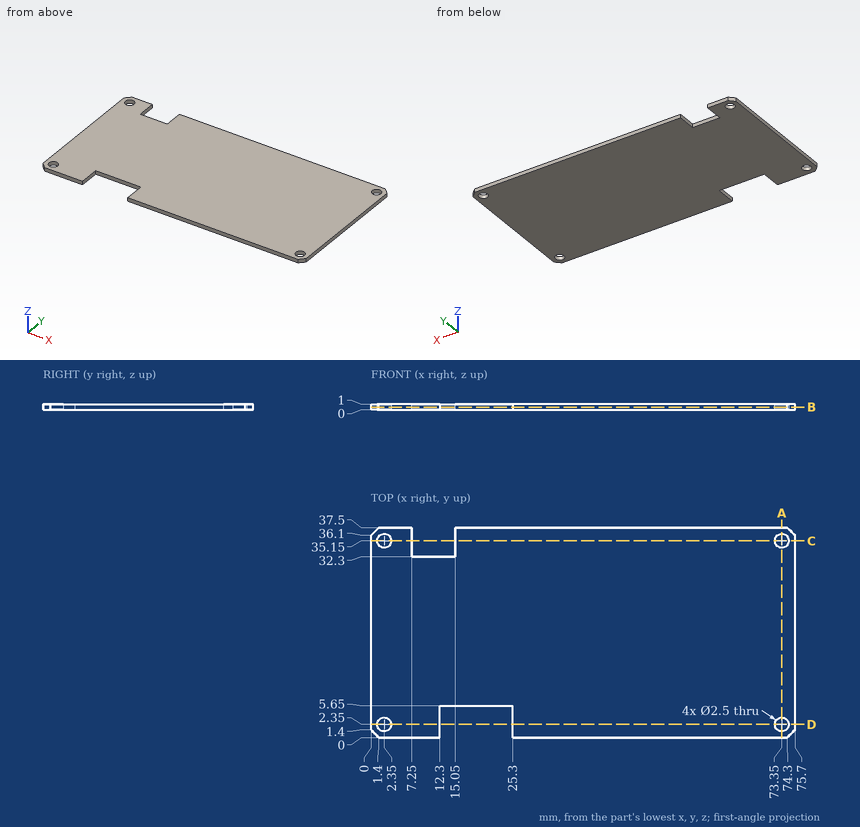
Verification items for this drawing (mm, ordinates from the low corner). Give positions to 0.01 mm unless a question says otherwise; leave off trailing zeros. Loops run counter-clockwise (first coordinate to the right, second up) from the corner with the lowest first, then second, coordinate; pieces in that order, holes last.
(1) Section check D-D on y = 2.35. Record the cut outline in (x, z).
From the geometry:
outline: (0, 0) - (1.1, 0) - (1.1, 1) - (0, 1) - close; (3.6, 0) - (12.3, 0) - (12.3, 1) - (3.6, 1) - close; (25.3, 0) - (72.1, 0) - (72.1, 1) - (25.3, 1) - close; (74.6, 0) - (75.7, 0) - (75.7, 1) - (74.6, 1) - close
(2) Depth check by flat-ended pin: pin 1 Ø10 at (x, y) = (54.5, 21.5) entering from -Z; pin 2 Ø0.5 at (x, z) = (9.5, 0.5) entering from +Y; pin 3 Ø1.5 at (x, y) = (73.35, 35.15) entering from -Z. Enter the tip coordinate at first touch or a pass-through.
From the geometry:
pin 1: stops at z = 0
pin 2: stops at y = 32.3
pin 3: passes through
(3) Section check A-A on x = 73.35. Record the cut outline in (y, z).
From the geometry:
outline: (0, 0) - (1.1, 0) - (1.1, 1) - (0, 1) - close; (3.6, 0) - (33.9, 0) - (33.9, 1) - (3.6, 1) - close; (36.4, 0) - (37.5, 0) - (37.5, 1) - (36.4, 1) - close
(4) Section check C-C on y = 35.15. Record the cut outline in (x, z).
From the geometry:
outline: (0, 0) - (1.1, 0) - (1.1, 1) - (0, 1) - close; (3.6, 0) - (7.25, 0) - (7.25, 1) - (3.6, 1) - close; (15.05, 0) - (72.1, 0) - (72.1, 1) - (15.05, 1) - close; (74.6, 0) - (75.7, 0) - (75.7, 1) - (74.6, 1) - close
(5) Section check B-B on z = 0.45. Record the cut outline in (x, y).
From the geometry:
outline: (0, 1.4) - (1.4, 0) - (12.3, 0) - (12.3, 5.65) - (25.3, 5.65) - (25.3, 0) - (74.3, 0) - (75.7, 1.4) - (75.7, 36.1) - (74.3, 37.5) - (15.05, 37.5) - (15.05, 32.3) - (7.25, 32.3) - (7.25, 37.5) - (1.4, 37.5) - (0, 36.1) - close; hole circle Ø2.5 at (2.35, 2.35); hole circle Ø2.5 at (2.35, 35.15); hole circle Ø2.5 at (73.35, 2.35); hole circle Ø2.5 at (73.35, 35.15)
(6) Thickness scan on L1, parallel to X at y = 2, z = 0.95; L2, parallel to Y at x = 12.5, z = 0.6; L3, parallel to Y at x = 19.5, z = 0.1. Record the ranges inside material, lowest first.
From the geometry:
L1: x = 0 to 1.15, 3.55 to 12.3, 25.3 to 72.15, 74.55 to 75.7
L2: y = 5.65 to 32.3
L3: y = 5.65 to 37.5
